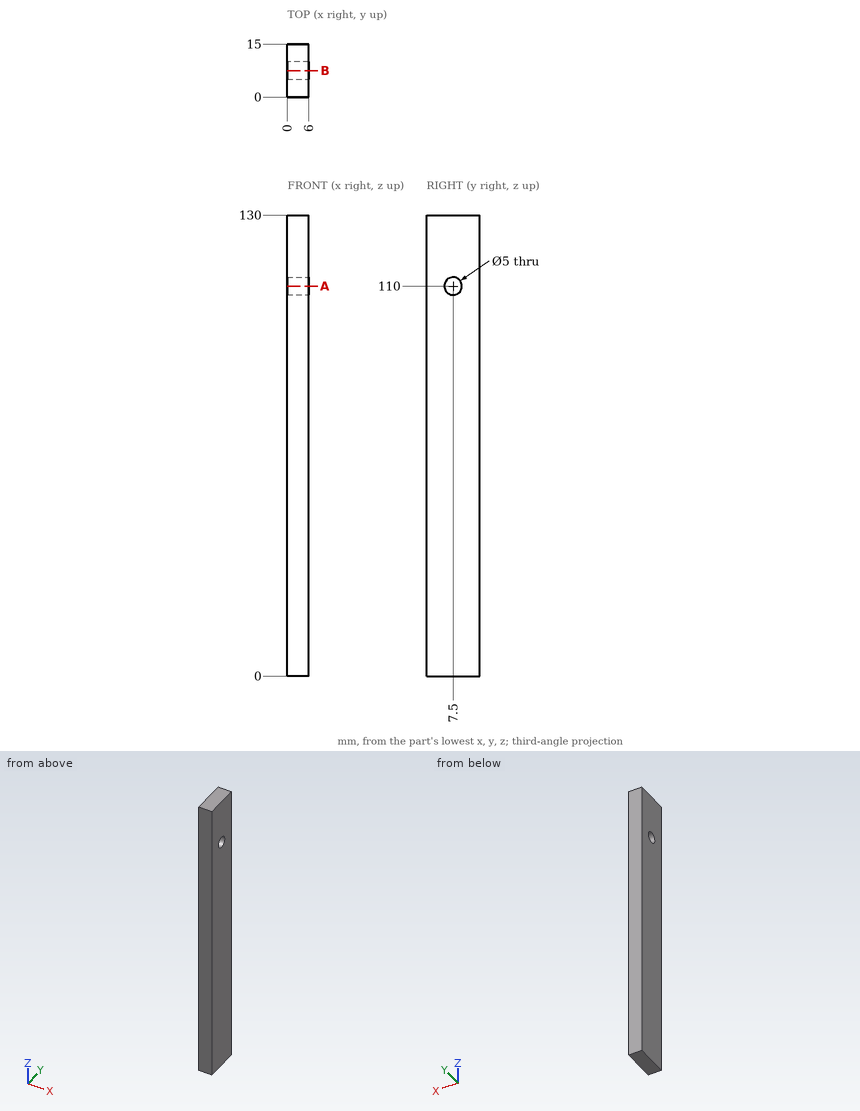
Here's the drawing with two shaded views (mm, measured from the low corner). I have some questions. Coordinates: 2 decimals unless noted, no trailing zeros. Loops run counter-clockwise (first coordinate to the right, second up) from the corner with the lowest first, then second, coordinate; pieces in that order, holes last. Notation, with made-up numbers: (-39.75, 78) - (0.25, 78) arc R10 cw to (0.25, 97) - close; hole circle Ø3 at (-30.5, 24.25). An arc over 180 degrees is marked (long way). Answer as CSV lines item,"result". Start each with the question number.
1) Suppose I cut it at B-B (y = 7.5). Please give me the cut outline in (x, z).
2) I need wall thicknesses on line 1 (Z direction, x = 1.65, y = 7.5); line 2 (Y direction, x = 4.55, z = 110); line 3 (Z direction, x = 3.05, y = 8.5). Which ranges of each line are inside material? Lowest first, please. Write a range as from..to.
3) Suppose I cut it at A-A (z = 110). Please give me the cut outline in (x, y), plus the area to 3 significant figures.
4) For pin 1 (3 mm diameter, centred on y = 7.5, z = 110, fed in from -X), with a flat end and sliding along its axis, tell me the tip position at first contact or that it passes through.
Check result:
1,outline,"(0, 0) - (6, 0) - (6, 107.5) - (0, 107.5) - close; (0, 112.5) - (6, 112.5) - (6, 130) - (0, 130) - close"
2,line 1,"z = 0..107.5, 112.5..130"
2,line 2,"y = 0..5, 10..15"
2,line 3,"z = 0..107.71, 112.29..130"
3,outline,"(0, 0) - (6, 0) - (6, 5) - (0, 5) - close; (0, 10) - (6, 10) - (6, 15) - (0, 15) - close"
3,area,"60.0 mm²"
4,pin 1,"passes through"
